Autodesk Inventor part; units mm, degrees
ref_plane "YZ Plane" through (0, 0, 0) normal (1, 0, 0) x (0, 1, 0)
ref_plane "XZ Plane" through (0, 0, 0) normal (0, 1, 0) x (-1, 0, 0)
ref_plane "XY Plane" through (0, 0, 0) normal (0, 0, 1) x (1, 0, 0)
sketch "Náčrt3" plane through (0, 0, 0) normal (0, 0, 1) x (1, 0, 0)
  line L0 (0, 0) -> (25, 0)
  line L1 (25, 0) -> (25, 55)
  line L2 (25, 55) -> (-15, 55)
  line L3 (-15, 55) -> (-15, 15)
  line L4 (-15, 15) -> (0, 15)
  line L5 (0, 15) -> (0, 0)
  dimension "d7" = 25
  dimension "d8" = 55
  dimension "d9" = 40
  dimension "d10" = 40
  dimension "d11" = 15
extrude "Vysunutí2" add sketch "Náčrt3" along normal blind 15
sketch "Náčrt4" plane through (0, 0, 15) normal (0, 0, 1) x (1, 0, 0)
  line L0 (25, 55) -> (-15, 55)
  line L1 (25, 55) -> (10, 55)
  line L2 (10, 55) -> (10, 40)
  line L3 (10, 40) -> (25, 40)
  line L4 (25, 40) -> (25, 55)
  point P0 (0, 0)
  dimension "d14" = 15
  dimension "d15" = 15
extrude "Vysunutí3" add sketch "Náčrt4" along normal blind 25
sketch "Náčrt5" plane through (-15, 55, 0) normal (0, 1, 0) x (1, 0, 0)
  point P0 (15, 0)
sketch "Náčrt6" plane through (-15, 55, 0) normal (0, 1, 0) x (1, 0, 0)
  line L0 (40, 0) -> (0, 0)
  line L1 (40, 0) -> (20, 0)
  line L2 (20, 0) -> (20, -10)
  line L3 (20, -10) -> (40, -10)
  line L4 (40, -10) -> (40, 0)
  point P0 (15, 0)
  dimension "d18" = 20
  dimension "d19" = 10
extrude "Vysunutí4" cut sketch "Náčrt6" against normal through all
properties part number "Součást1"
For this review, take the finished solid that the model builds, in its own axes (mm). A direction names the side the tool comes from. Round coordinates to 2 decimals unless told otherwise and drop trailing zeros. Write each loop counter-clockwise with the first axis right and the second up, starting at its lowest first coordinate (ties: lowest second). Pieces come first, ordered by that corner, then holes.
1) Take a section at B-B on x = 14.5. Give the boundary of the cut face in (y, z).
Answer below:
outline: (0, 10) - (55, 10) - (55, 40) - (40, 40) - (40, 15) - (0, 15) - close
2) Take a section at D-D on z = 31. Give the boundary of the cut face in (x, y).
Answer below:
outline: (10, 40) - (25, 40) - (25, 55) - (10, 55) - close
3) Take a section at C-C on x = 8.5. Give the boundary of the cut face in (y, z).
Answer below:
outline: (0, 10) - (55, 10) - (55, 15) - (0, 15) - close
4) For line 1 along X through (y, z) = (34, 4); line 2 along Z through (x, y) = (3, 32); line 3 along X through (y, z) = (11, 14.5), list the stretches that pass through material, from the lowest coordinate up.
Answer below:
line 1: x = -15 to 5
line 2: z = 0 to 15
line 3: x = 0 to 25
5) Take a section at A-A on z = 12.5. Give the boundary of the cut face in (x, y).
Answer below:
outline: (-15, 15) - (0, 15) - (0, 0) - (25, 0) - (25, 55) - (-15, 55) - close
6) Insertion check: pin 1 Ø7.5 at (y, z) = (47, 29.5) entering from -X; pin 2 Ø12 at (y, z) = (5.5, 4) entering from -X; pin 3 Ø16 at (x, y) = (11.5, 29.5) entering from -Z; pin 4 Ø12 at (x, y) = (1.5, 31.5) entering from +Z. Each pin has a flat end and moves straight along its axis. Give the tip position at first contact, or say it passes through.
Answer below:
pin 1: stops at x = 10
pin 2: stops at x = 0
pin 3: stops at z = 0
pin 4: stops at z = 15
7) Machinability: for faces 1 (the face through (17, 40, 27)), 2 (the face through (10, 48, 27)), 3 (the face through (5, 28, 5)), which of the approach directions +Z, -Z, +X, -X, +Y, -Y give a long, thin tool a straight path to every point of the face, cutting with its end or side? Answer none if there is none.
Answer below:
face 1: +Z, +X, -X, -Y
face 2: +Z, -X, +Y, -Y
face 3: -Z, +X, +Y, -Y
